```python
from build123d import *

# Parameters (mm, degrees)
BOSS_EXTRUDE1_DEPTH = 3
BOSS_EXTRUDE2_DEPTH = 3
SKETCH3_W           = 87.73773678
SKETCH3_H           = 3.000342445
CUT_EXTRUDE1_DEPTH  = 300


with BuildPart() as part:
    # Sketch1 → Boss-Extrude1 (new body)
    with BuildSketch(Plane.XY):
        with BuildLine():
            Line((93.97826087, 269), (101.804347826, 293))
            Line((101.804347826, 293), (20.086056782, 293))
            ThreePointArc((20.086056782, 293), (-7.9185527, 290.707315192), (-21.3, 266))
            Line((-21.3, 266), (-21.3, -5))
            Line((-21.3, -5), (0, -5))
            Line((0, -5), (0, 269))
            Line((0, 269), (93.97826087, 269))
        make_face()
    extrude(amount=BOSS_EXTRUDE1_DEPTH)

    # Sketch2 → Boss-Extrude2 (add)
    with BuildSketch(Plane.XY.offset(3)):
        Polygon((8.199539928, 295.500342445), (95.938079236, 295.500342445), (95.938079236, 293), (8.804994825, 293), align=None)
    extrude(amount=-BOSS_EXTRUDE2_DEPTH)

    # Sketch3 → Cut-Extrude1 (cut)
    with BuildSketch(Plane(origin=(0, 0, 0), x_dir=(-1, 0, 0), z_dir=(0, 0, -1))):
        with Locations((-52.069210846, 294.000171223)):
            Rectangle(SKETCH3_W, SKETCH3_H)
    extrude(amount=-CUT_EXTRUDE1_DEPTH, mode=Mode.SUBTRACT)


solid = part.part
```
Can you work these out from the model? Positions are in its coordinate system, mm. Coordinates: 2 decimals unless noted, no trailing zeros. Loops run counter-clockwise (first coordinate to the right, second up) from the corner with the lowest first, then second, coordinate; pieces in that order, holes last.
Item 1: Suppose I cut it at B-B (x = 82). Please give me the cut outline in (y, z).
Answers below:
outline: (269, 0) - (292.5, 0) - (292.5, 3) - (269, 3) - close
Item 2: I'm going to push flat-ended pins straight in: pin 1 (1.5 mm diameter, centred on x = 45, z = 2, fed in from -Y); pin 2 (0.9 mm diameter, centred on x = 47.5, z = 1, fed in from +Y); pin 3 (0.9 mm diameter, centred on y = 173.5, z = 1.5, fed in from +X). Where does each tip first touch, or does it pass through?
Answers below:
pin 1: stops at y = 269
pin 2: stops at y = 292.5
pin 3: stops at x = 0
Item 3: Please list where these lines run through material, in increasing order: L1, parallel to Y at x = 75, z = 1.7; L2, parallel to X at y = 76.5, z = 0.9; L3, parallel to X at y = 271.5, z = 2.
Answers below:
L1: y = 269 to 292.5
L2: x = -21.3 to 0
L3: x = -20.78 to 94.79
Item 4: Suppose I cut it at C-C (y = 115). Please give me the cut outline in (x, z).
Answers below:
outline: (-21.3, 0) - (0, 0) - (0, 3) - (-21.3, 3) - close
Item 5: Suppose I cut it at A-A (z = 0.65). Please give me the cut outline in (x, y).
Answers below:
outline: (-21.3, -5) - (0, -5) - (0, 269) - (93.98, 269) - (101.8, 293) - (95.94, 293) - (95.94, 292.5) - (8.2, 292.5) - (8.2, 295.5) arc R29.5 ccw to (-21.3, 266) - close
